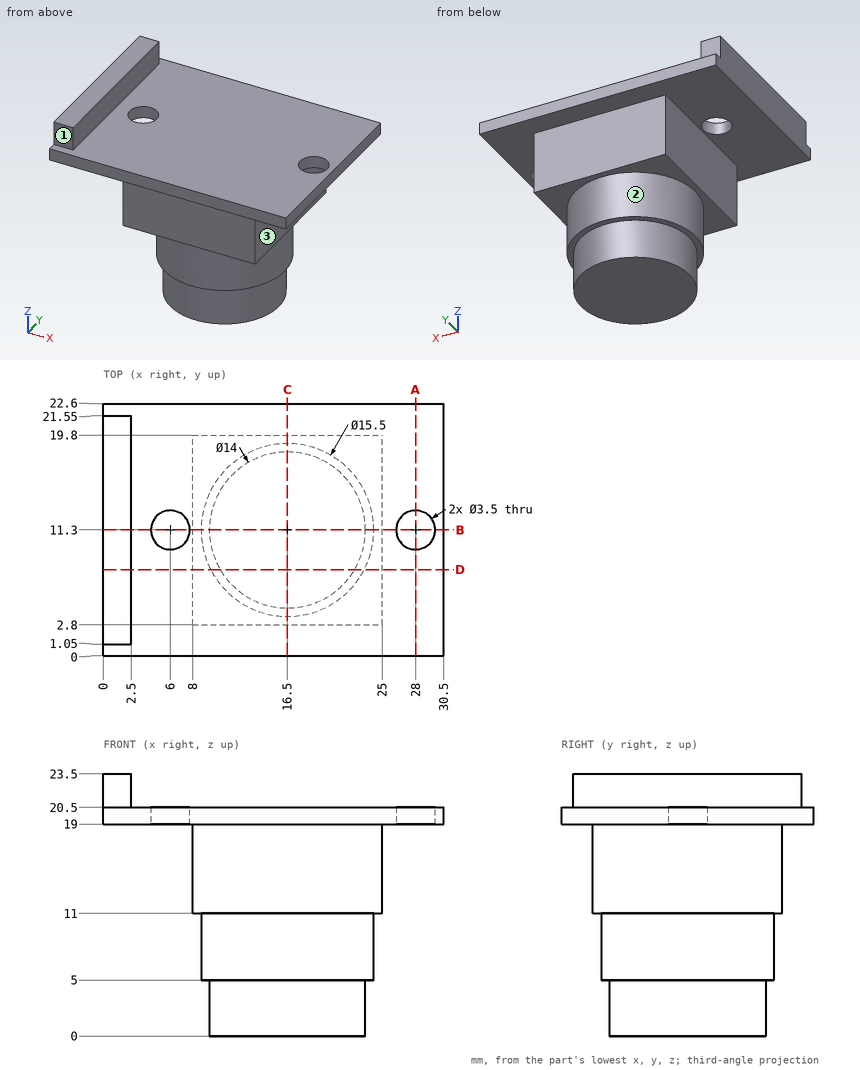
Design review of the part shown in the three views and the two pictorial views. Dimensions are in mm from the part's minimum x, y and z. A direction names the side the tool comes from. Give positions to 0.01 mm unless a question says otherwise; leave off trailing zeros. Loops run counter-clockwise (first coordinate to the right, second up) from the corner with the lowest first, then second, coordinate; pieces in that order, holes last. Notation, with made-up numbers: (-2.75, 12) -> (38.25, 12) arc R34 cw to (38.25, 48) -> close; hole circle Ø5 at (-23, -8.5). An arc over 180 degrees is marked (long way). Write each question's results on one line, items separated by ' | '.
Q1. Machinability: for the marked faces 1, 2 and 3, which of the approach directions +Z, -Z, +X, -X, +Y, -Y give a long, thin tool a straight path to every point of the face, cutting with its end or side? Answer none if there is none.
Reply:
face 1: +Z, +X, -X, -Y | face 2: -Z | face 3: -Z, +X, +Y, -Y
Q2. Take a section at B-B, the plane y = 11.3. Write out the cut boundary in (x, z).
Reply:
outline: (0, 19) -> (4.25, 19) -> (4.25, 20.5) -> (2.5, 20.5) -> (2.5, 23.5) -> (0, 23.5) -> close; (7.75, 19) -> (8, 19) -> (8, 11) -> (8.75, 11) -> (8.75, 5) -> (9.5, 5) -> (9.5, 0) -> (23.5, 0) -> (23.5, 5) -> (24.25, 5) -> (24.25, 11) -> (25, 11) -> (25, 19) -> (26.25, 19) -> (26.25, 20.5) -> (7.75, 20.5) -> close; (29.75, 19) -> (30.5, 19) -> (30.5, 20.5) -> (29.75, 20.5) -> close
Q3. Wall thickness on L1, parallel to Y at x = 28, z = 19.6; L2, parallel to Z at x = 17.5, y = 6.75; L3, parallel to X at y = 12, z = 15.5: over which ranges is each line inside the solid? List them lowest first.
Reply:
L1: y = 0 to 9.55, 13.05 to 22.6 | L2: z = 0 to 20.5 | L3: x = 8 to 25
Q4. For pin 1 Ø2 at (x, z) = (0.5, 22.5) entering from -Y; pin 2 Ø1.5 at (x, z) = (25.5, 4) entering from +Y; pin 3 Ø3 at (x, z) = (25.5, 16) entering from -Y; pin 4 Ø5.5 at (x, y) = (6, 11.3) entering from +Z, all flat-tipped, find the tip position at first contact; note any pin that passes through.
Reply:
pin 1: stops at y = 1.05 | pin 2: passes through | pin 3: stops at y = 2.8 | pin 4: stops at z = 20.5
Q5. Take a section at A-A, the plane x = 28. Write out the cut boundary in (y, z), plus the area to 4 significant figures.
Reply:
outline: (0, 19) -> (9.55, 19) -> (9.55, 20.5) -> (0, 20.5) -> close; (13.05, 19) -> (22.6, 19) -> (22.6, 20.5) -> (13.05, 20.5) -> close | area: 28.65 mm²
Q6. Take a section at C-C, the plane x = 16.5. Write out the cut boundary in (y, z).
Reply:
outline: (0, 19) -> (2.8, 19) -> (2.8, 11) -> (3.55, 11) -> (3.55, 5) -> (4.3, 5) -> (4.3, 0) -> (18.3, 0) -> (18.3, 5) -> (19.05, 5) -> (19.05, 11) -> (19.8, 11) -> (19.8, 19) -> (22.6, 19) -> (22.6, 20.5) -> (0, 20.5) -> close
Q7. Take a section at D-D, the plane y = 7.75. Write out the cut boundary in (x, z).
Reply:
outline: (0, 19) -> (8, 19) -> (8, 11) -> (9.61, 11) -> (9.61, 5) -> (10.47, 5) -> (10.47, 0) -> (22.53, 0) -> (22.53, 5) -> (23.39, 5) -> (23.39, 11) -> (25, 11) -> (25, 19) -> (30.5, 19) -> (30.5, 20.5) -> (2.5, 20.5) -> (2.5, 23.5) -> (0, 23.5) -> close
